Source: CAD feature listing. Evaluate the final solid. Frame: model axes, mm. Give positions to 0.01 mm unless a question says otherwise; leave off trailing zeros. Write each loop counter-clockwise with the first axis right and the second up, starting at its lowest first coordinate (ties: lowest second). Pieces come first, ordered by that corner, then holes. Notation, with made-up numbers: (18.5, 49.5) -> (27.5, 49.5) arc R13 cw to (27.5, 57.5) -> close; hole circle Ø4 at (81, -16). An arc over 180 degrees is marked (long way). Use one line per item in the form item = value. Start each with the question number.
(1) Cut plane A-A, the plane x = 18.5. Output: boundary loops of the cut face in (y, z), and give its area (3 significant figures).
(2) First-contact query: P1, Ø2, axis at x = 58.5, y = 11, coming from the +Z side; P2, Ø1, axis at y = 3, z = 74.5, coming from the +X side. Flat tips, straight axial feed; report the tip coordinate or a pass-through.
(3) Material intervals for line 1 along Y through (x, z) = (65.5, 71); line 2 along X through (y, z) = (4.75, 39); line 3 along Y through (x, z) = (67.5, 114.5), sorted ascending. Write a range as from..to.
from build123d import *

# Parameters (mm, degrees)
ESQUISSE1_W             = 70
ESQUISSE1_H             = 25
BOSS_EXTRU_1_DEPTH      = 150
CONG_1_R                = 5
ESQUISSE2_W             = 13
ESQUISSE2_H             = 7
ESQUISSE2_W_2           = 10
ESQUISSE2_H_2           = 2.5
ENL_V_MAT_EXTRU_1_DEPTH = 11.5


with BuildPart() as part:
    # Esquisse1 → Boss.-Extru.1 (new body)
    with BuildSketch(Plane.XY):
        with Locations((35, 12.5)):
            Rectangle(ESQUISSE1_W, ESQUISSE1_H)
    extrude(amount=BOSS_EXTRU_1_DEPTH)

    # Congé1
    cong_1_edges = [part.edges().sort_by_distance(p)[0] for p in [
        (0, 25, 75),
        (70, 25, 75),
        (70, 0, 75),
        (0, 0, 75),
    ]]
    fillet(cong_1_edges, radius=CONG_1_R)

    # Esquisse2 → Enlèv. mat.-Extru.1 (cut)
    with BuildSketch(Plane.XY.offset(150)):
        with Locations((14.5, 12.5)):
            Rectangle(ESQUISSE2_W, ESQUISSE2_H)
        with Locations((55.5, 12.5)):
            Rectangle(ESQUISSE2_W, ESQUISSE2_H)
        with Locations((35, 12.75)):
            Rectangle(ESQUISSE2_W_2, ESQUISSE2_H_2)
    extrude(amount=-ENL_V_MAT_EXTRU_1_DEPTH, mode=Mode.SUBTRACT)


solid = part.part
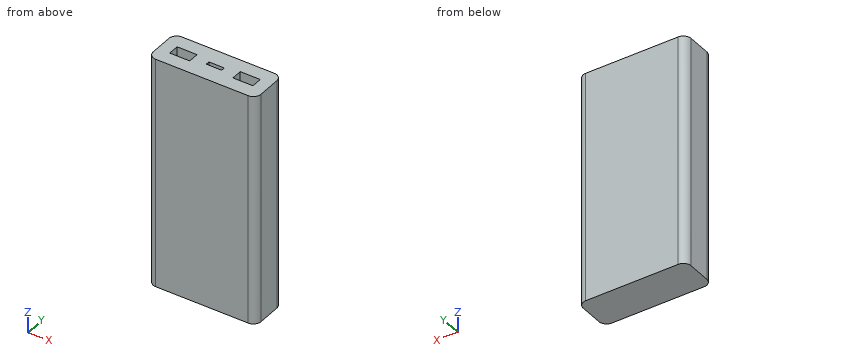
Geometry says:
q1.outline = (0, 0) -> (25, 0) -> (25, 150) -> (16, 150) -> (16, 138.5) -> (9, 138.5) -> (9, 150) -> (0, 150) -> close
q1.area = 3,670 mm^2
q2.P1 = 138.5
q2.P2 = 69.77
q3.line_1 = 0.03..24.97
q3.line_2 = 0.01..69.99
q3.line_3 = 0.67..24.33
